Source: CAD feature listing. Evaluate the final solid. Frame: model axes, mm. Face numbers are marked on the shaded views. Give positions to 0.01 mm unless a question says otherwise; leave off trailing zeros.
Autodesk Inventor part; units mm, degrees
ref_plane "YZ Plane" through (0, 0, 0) normal (1, 0, 0) x (0, 1, 0)
ref_plane "XZ Plane" through (0, 0, 0) normal (0, 1, 0) x (-1, 0, 0)
ref_plane "XY Plane" through (0, 0, 0) normal (0, 0, 1) x (1, 0, 0)
sketch "Sketch1" plane through (0, 0, 0) normal (0, 0, 1) x (1, 0, 0)
  line L0 (37.5, -37.5) -> (-37.5, -37.5)
  line L1 (-37.5, -37.5) -> (-37.5, 37.5)
  line L2 (-37.5, 37.5) -> (37.5, 37.5)
  line L3 (37.5, 37.5) -> (37.5, -37.5)
  line L4 (37.5, -37.5) -> (-37.5, 37.5) construction
  line L5 (-37.5, -37.5) -> (37.5, 37.5) construction
  line L6 (32.5, 32.5) -> (-32.5, 32.5)
  line L7 (-32.5, 32.5) -> (-32.5, -32.5)
  line L8 (-32.5, -32.5) -> (32.5, -32.5)
  line L9 (32.5, -32.5) -> (32.5, 32.5)
  line L10 (32.5, 32.5) -> (-32.5, -32.5) construction
  line L11 (-32.5, 32.5) -> (32.5, -32.5) construction
  line L12 (30.5, 30.5) -> (-30.5, 30.5)
  line L13 (-30.5, 30.5) -> (-30.5, -30.5)
  line L14 (-30.5, -30.5) -> (30.5, -30.5)
  line L15 (30.5, -30.5) -> (30.5, 30.5)
  line L16 (30.5, 30.5) -> (-30.5, -30.5) construction
  line L17 (-30.5, 30.5) -> (30.5, -30.5) construction
  line L18 (-4.8636, 37.5) -> (-36.3868, 37.5)
  line L19 (0, 41.9833) -> (-15.7401, 41.9833)
  line L20 (-15.7401, 41.9833) -> (-15.7401, 37.5)
  line L21 (0, 41.9833) -> (15.8927, 41.9833)
  line L22 (15.8927, 41.9833) -> (15.8927, 37.5)
  point P0 (0, 0)
  dimension "d2" = 65
  dimension "d3" = 65
  dimension "d4" = 2
  dimension "d5" = 2
  dimension "d22" = 5
  dimension "d23" = 5
extrude "Extrusion1" add sketch "Sketch1" along normal blind 3 contours L0 L1 L2 L3 | L2 L20 L19 L21 L22 | L9 L8 L7 L6 | L15 L14 L13 L12
extrude "Extrusion2" add sketch "Sketch1" against normal blind 5 contours L9 L8 L7 L6
chamfer "Chamfer1" distance 1.5875 angle 45 8 edges at (0, -37.5, 3) (-37.5, 0, 3) (26.6963, 37.5, 3) (-26.62, 37.5, 3) (37.5, 0, 3) (15.8927, 39.7416, 3) (0.0763, 41.9833, 3) (-15.7401, 39.7416, 3)
fillet "Fillet2" radius 3.175 8 edges at (-37.5, -37.5, 0.7063) (37.5, -37.5, 0.7063) (37.5, 37.5, 0.7063) (-37.5, 37.5, 0.7063) (15.8927, 37.5, 0.7063) (15.8927, 41.9833, 0.7063) (-15.7401, 41.9833, 0.7063) (-15.7401, 37.5, 0.7063)
thicken "Thicken1" operation cut thickness 0.125 both sides no extend neighbours no toward (1, 0, 0) faces at (-32.5, 10.8333, -3.3333) (-10.8333, -32.5, -3.3333) (32.5, -10.8333, -3.3333) (10.8333, 32.5, -3.3333)
fillet "Fillet3" radius 1.5875 4 edges at (32.375, 0, -5) (-32.375, 0, -5) (0, 32.375, -5) (0, -32.375, -5)
properties part number "Lid" material "PET Plastic"
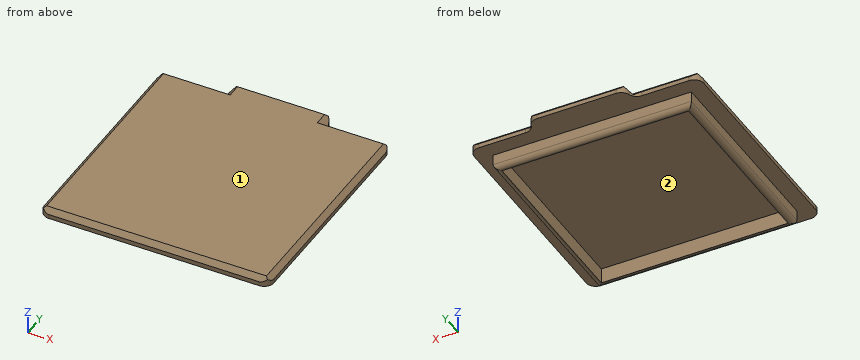
1. Mould query, pull axis Y, two halves, no side actions, for the marked faces 1 and 2. Classes: +Y half, -Y half, draft (parallel to the pull), parting line (faces both ways), or undercut.
2. Line query: L1, parallel to Y at x = 7.5, z = -2.75 (3 decimals); L2, parallel to Z at x = -4.5, y = 6. Output: solid intervals per line, ascending.
3. Contact query for flat-ended pins moving along their axis: P1, Ø12, axis at x = -15.5, y = 3.5, coming from the -Z side; P2, Ø4, axis at y = -11.5, z = -2.5, coming from the -X side (3 decimals); P3, Ø2.5, axis at x = 7, z = -2, coming from the -Y side (3 decimals). Output: stop coordinate, or through.
Response values:
1. face 1: draft
1. face 2: undercut
2. L1: y = -32.375 to -30.5, 30.5 to 32.375
2. L2: z = 0 to 3
3. P1: stops at z = 0
3. P2: stops at x = -32.375
3. P3: stops at y = -32.375
